Work out the finished part from the listing and answer in its coordinate system (mm). Face numbers are marked on the shaded views. A direction names the side the tool comes from. Round coordinates to 2 decimals unless told otherwise and drop trailing zeros. Loops run counter-clockwise (first coordinate to the right, second up) from the corner with the lowest first, then second, coordinate; pieces in that order, holes last. Notation, with made-up numbers: (27, 30) - (68, 30) arc R13 cw to (68, 52) - close; hole circle Ø2 at (10, -25). An arc over 180 degrees is marked (long way). Answer as CSV lines item,"result". Start each with the question number.
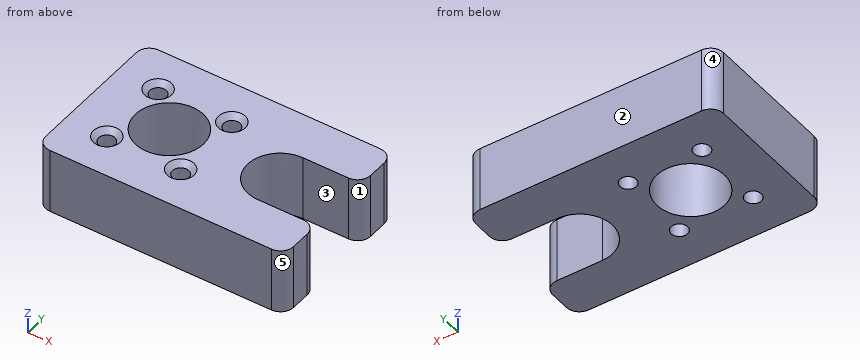
```python
from build123d import *

# Parameters (mm, degrees)
F0_R     = 1.25
F0_R_2   = 5.2
F1_DEPTH = 10
F2_R     = 2
F3_SIZE  = 0.8


with BuildPart() as f1:
    # F0 (on Top) → F1 (new body)
    with BuildSketch(Plane.XY):
        with BuildLine():
            Line((19, 5), (19, 12))
            Line((19, 12), (-19, 12))
            Line((-19, 12), (-19, -12))
            Line((-19, -12), (19, -12))
            Line((19, -12), (19, -5))
            Line((19, -5), (10, -5))
            ThreePointArc((10, -5), (5, 0), (10, 5))
            Line((10, 5), (19, 5))
        make_face()
        with Locations((-12.656854, -5.656854)):
            Circle(F0_R, mode=Mode.SUBTRACT)
        with Locations((-1.343146, -5.656854)):
            Circle(F0_R, mode=Mode.SUBTRACT)
        with Locations((-12.656854, 5.656854)):
            Circle(F0_R, mode=Mode.SUBTRACT)
        with Locations((-7, 0)):
            Circle(F0_R_2, mode=Mode.SUBTRACT)
        with Locations((-1.343146, 5.656854)):
            Circle(F0_R, mode=Mode.SUBTRACT)
    extrude(amount=F1_DEPTH)

    # F2
    f2_edges = [f1.edges().sort_by_distance(p)[0] for p in [
        (-19, -12, 5),
        (-19, 12, 5),
        (19, -12, 5),
        (19, -5, 5),
        (19, 5, 5),
        (19, 12, 5),
    ]]
    fillet(f2_edges, radius=F2_R)

    # F3
    f3_edges = [f1.edges().sort_by_distance(p)[0] for p in [
        (-13.906854, 5.656854, 10),
        (-2.593146, 5.656854, 10),
        (-2.593146, -5.656854, 10),
        (-13.906854, -5.656854, 10),
    ]]
    chamfer(f3_edges, length=F3_SIZE)


solid = f1.part
```
Item 1: Section C-C, the plane z = 1.75 is taken. Give the vertices of the cut face in (x, y).
Item 2: Section B-B, the plane y = 0 is taken. Give the vertices of the cut face in (x, z), and give its area (3 significant figures).
Item 3: Section A-A, the plane x = -7 is taken. Give the vertices of the cut face in (y, z).
Item 4: Which of the six approach directions +Z, -Z, +X, -X, +Y, -Y give full straight-line access (tool end or side, diameter ignored) to the marked faces 1 and 2?
Item 5: A flat-ended cylindrical pin translates along its axis: pin 1 Ø4 at (x, y) = (-12.66, 5.66) entering from +Z. Find the tip coordinate at first contact, or state that the pin passes through.
Item 6: Find the intervals of material crossed by L1, parallel to X at y = 6.25, z = 4; L2, parallel to X at y = -0.25, z = 2.75; L3, parallel to Y at x = -7, z = 3.75, in increasing order.
Item 7: Determine the mould class of the marked faces 3, 4 and 5 for opening direction Y: pulls with the +Y half, pulls with the -Y half, needs draft (parallel to the pull), parting line crosses it, or undercut.
Answer:
1,outline,"(-19, -10) arc R2 ccw to (-17, -12) - (17, -12) arc R2 ccw to (19, -10) - (19, -7) arc R2 ccw to (17, -5) - (10, -5) arc R5 cw to (10, 5) - (17, 5) arc R2 ccw to (19, 7) - (19, 10) arc R2 ccw to (17, 12) - (-17, 12) arc R2 ccw to (-19, 10) - close; hole circle Ø2.5 at (-12.66, -5.66); hole circle Ø2.5 at (-12.66, 5.66); hole circle Ø10.4 at (-7, 0); hole circle Ø2.5 at (-1.34, -5.66); hole circle Ø2.5 at (-1.34, 5.66)"
2,outline,"(-19, 0) - (-12.2, 0) - (-12.2, 10) - (-19, 10) - close; (-1.8, 0) - (5, 0) - (5, 10) - (-1.8, 10) - close"
2,area,"136 mm²"
3,outline,"(-12, 0) - (-5.2, 0) - (-5.2, 10) - (-12, 10) - close; (5.2, 0) - (12, 0) - (12, 10) - (5.2, 10) - close"
4,face 1,"+Z, -Z, +X"
4,face 2,"+Z, -Z, +X, -X, +Y"
5,pin 1,"stops at z = 9.95"
6,L1,"x = -19 to -13.76, -11.56 to -2.44, -0.24 to 18.85"
6,L2,"x = -19 to -12.19, -1.81 to 5.01"
6,L3,"y = -12 to -5.2, 5.2 to 12"
7,face 3,"undercut"
7,face 4,"pulls with the +Y half"
7,face 5,"pulls with the -Y half"
